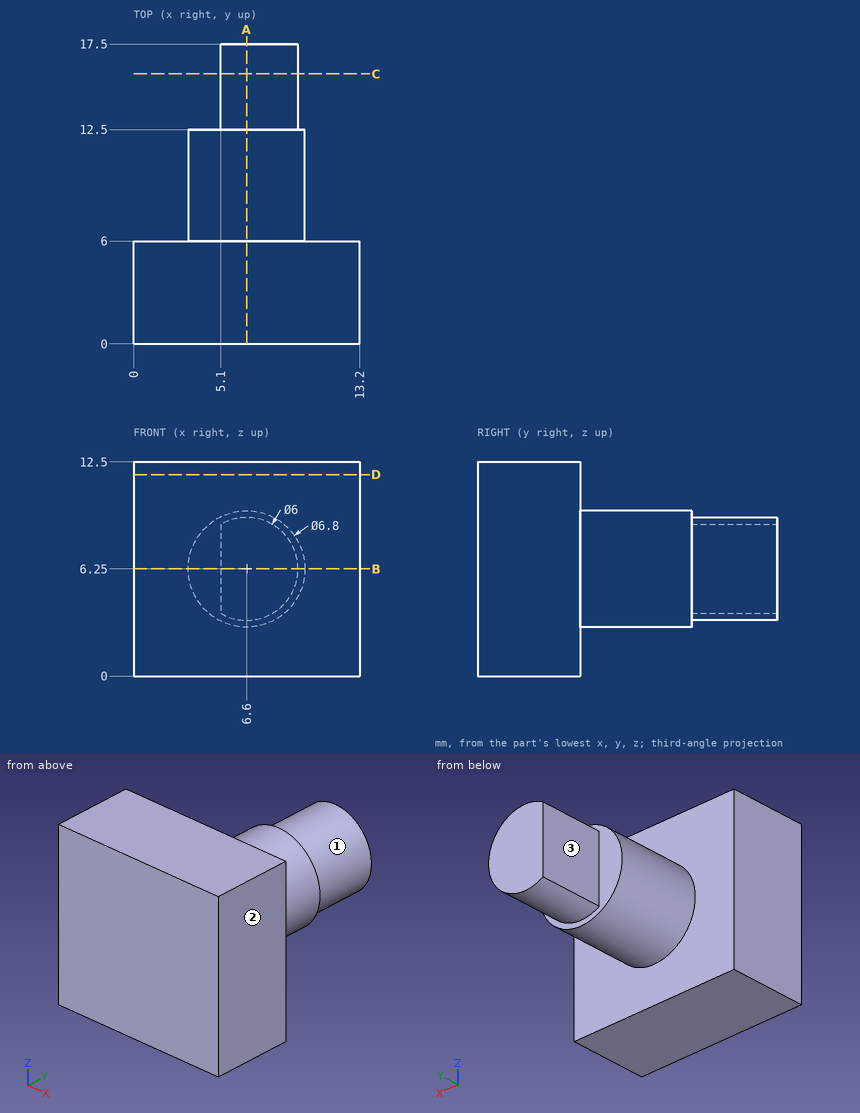
Input: dimensioned drawing with shaded views. Units: mm. Origin: part minimum x, y, z. A direction names the side the tool comes from. Round coordinates to 2 decimals unless told otherwise and drop trailing zeros. Loops run counter-clockwise (first coordinate to the right, second up) from the corner with the lowest first, then second, coordinate; pieces in that order, holes last. Notation, with made-up numbers: M -22,14.5 L 16,14.5 A34 cw 16,50.5 Z; hole C 28,63.25 d6. An arc over 180 degrees is marked long. Return JSON: item names as keys, results as strings. Group by question number.
1. Section query B-B on z = 6.25. Output: boundary loops of the cut face in (x, y), and give its area (3 significant figures).
2. Section query C-C on y = 15.75. Output: boundary loops of the cut face in (x, z), and give its area (3 significant figures).
3. Pin query (flat end, axial travel): pin 1 (1.5 mm diameter, centred on y = 14.5, z = 6.5, fed in from -X); pin 2 (4 mm diameter, centred on y = 13.5, z = 4.5, fed in from -X); pin 3 (1.5 mm diameter, centred on y = 13, z = 3, fed in from +X). Return the tip coordinate at first contact, or that it passes through.
4. Section query D-D on z = 11.75. Output: boundary loops of the cut face in (x, y), and give its area (3 significant figures).
5. Reachability of the marked faces 1, 2 and 3 from +Z, -Z, +X, -X, +Y, -Y: full face, straight path, thin tool, end or side. Return the list, or none.
6. Section query A-A on x = 6.6. Output: boundary loops of the cut face in (y, z).
7. Material intervals for line 1 along Y through (x, z) = (1.25, 6.25); line 2 along Z through (x, y) = (8.75, 7.5); line 3 along Z through (x, y) = (6.5, 16), sorted ascending. Write a range as from..to.
Checks:
{
 "1": {"outline": "M 0,0 L 13.2,0 L 13.2,6 L 10,6 L 10,12.5 L 9.6,12.5 L 9.6,17.5 L 5.1,17.5 L 5.1,12.5 L 3.2,12.5 L 3.2,6 L 0,6 Z", "area": "146 mm²"},
 "2": {"outline": "M 5.1,3.65 A3 ccw long 5.1,8.85 Z", "area": "22.7 mm²"},
 "3": {"pin 1": "stops at x = 5.1", "pin 2": "stops at x = 3.2", "pin 3": "stops at x = 8.68"},
 "4": {"outline": "M 0,0 L 13.2,0 L 13.2,6 L 0,6 Z", "area": "79.2 mm²"},
 "5": {"face 1": "+Y", "face 2": "+Z, -Z, +X, +Y, -Y", "face 3": "+Z, -Z, -X, +Y"},
 "6": {"outline": "M 0,0 L 6,0 L 6,2.85 L 12.5,2.85 L 12.5,3.25 L 17.5,3.25 L 17.5,9.25 L 12.5,9.25 L 12.5,9.65 L 6,9.65 L 6,12.5 L 0,12.5 Z"},
 "7": {"line 1": "y = 0..6", "line 2": "z = 3.62..8.88", "line 3": "z = 3.25..9.25"}
}
